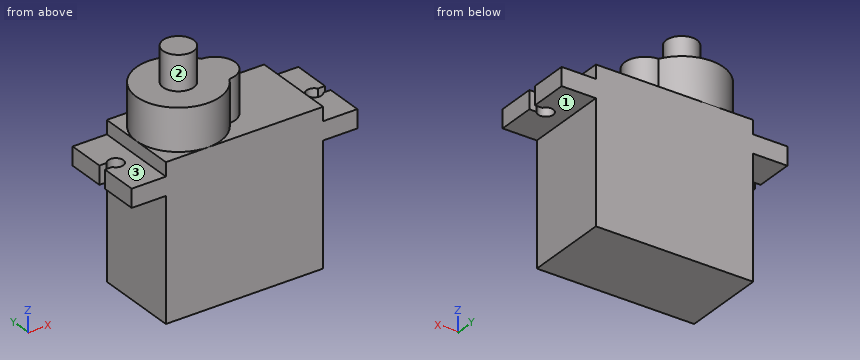
```python
from build123d import *

# Parameters (mm, degrees)
SKETCH2_W           = 23
SKETCH2_H           = 12.3
BOSS_EXTRUDE1_DEPTH = 22.4
SKETCH3_W           = 2.67
SKETCH3_H           = 12.3
BOSS_EXTRUDE2_DEPTH = 5
CUT_EXTRUDE1_DEPTH  = 27.948701267
BOSS_EXTRUDE3_DEPTH = 6.13
SKETCH5_R           = 2.25
BOSS_EXTRUDE4_DEPTH = 5.05


with BuildPart() as part:
    # Sketch2 → Boss-Extrude1 (new body)
    with BuildSketch(Plane.XY):
        Rectangle(SKETCH2_W, SKETCH2_H)
    extrude(amount=BOSS_EXTRUDE1_DEPTH)

    # Sketch3 → Boss-Extrude2 (add)
    with BuildSketch(Plane(origin=(11.5, 0, 0), x_dir=(0, 0, -1), z_dir=(1, 0, 0))):
        with Locations((-19.065, 0)):
            Rectangle(SKETCH3_W, SKETCH3_H)
    boss_extrude2 = extrude(amount=BOSS_EXTRUDE2_DEPTH)

    # Sketch6 → Cut-Extrude1 (cut, through all)
    with BuildSketch(Plane.XY.offset(20.4)):
        with BuildLine():
            Line((15.437749967, 0.575), (16.5, 0.575))
            Line((16.5, 0.575), (16.5, -0.575))
            Line((16.5, -0.575), (15.437749967, -0.575))
            ThreePointArc((15.437749967, -0.575), (13.4, 0), (15.437749967, 0.575))
        make_face()
    cut_extrude1 = extrude(amount=-CUT_EXTRUDE1_DEPTH, mode=Mode.SUBTRACT)

    # Mirror1: Boss-Extrude2, Cut-Extrude1 across plane
    add(boss_extrude2.mirror(Plane(origin=(0, 0, 0), x_dir=(0, 0, 1), z_dir=(1, 0, 0))))
    add(cut_extrude1.mirror(Plane(origin=(0, 0, 0), x_dir=(0, 0, 1), z_dir=(1, 0, 0))), mode=Mode.SUBTRACT)

    # Sketch4 → Boss-Extrude3 (add)
    with BuildSketch(Plane.XY.offset(22.4)):
        with BuildLine():
            ThreePointArc((0.060221963, 2.924379988), (-11.5, 0), (0.060221963, -2.924379988))
            ThreePointArc((0.060221963, -2.924379988), (2.925, 0), (0.060221963, 2.924379988))
        make_face()
    extrude(amount=BOSS_EXTRUDE3_DEPTH)

    # Sketch5 → Boss-Extrude4 (add)
    with BuildSketch(Plane.XY.offset(28.53)):
        with Locations((-5.35, 0)):
            Circle(SKETCH5_R)
    extrude(amount=BOSS_EXTRUDE4_DEPTH)


solid = part.part
```
Input: part model. Units: mm. Frame: model coordinates. Face numbers are marked on the shaded views. A direction names the side the tool comes from. Coordinates: 2 decimals unless noted, no trailing zeros. Loops run counter-clockwise (first coordinate to the right, second up) from the corner with the lowest first, then second, coordinate; pieces in that order, holes last.
Q1. Section D-D, the plane z = 2.5. Return the cut outline in (x, y).
Results are:
outline: (-11.5, -6.15) - (11.5, -6.15) - (11.5, 6.15) - (-11.5, 6.15) - close
Q2. Line query: line 1 along Y through (x, z) = (-14.5, 18.3); line 2 along Z through (x, y) = (-9.5, 1.25); line 3 along X through (y, z) = (0, 18.75). Output: solid intervals per line, ascending.
Results are:
line 1: y = -6.15 to -1.1, 1.1 to 6.15
line 2: z = 0 to 28.53
line 3: x = -13.4 to 13.4
Q3. Section B-B, the plane y = -4. Return the cut outline in (x, z).
Results are:
outline: (-16.5, 17.73) - (-11.5, 17.73) - (-11.5, 0) - (11.5, 0) - (11.5, 17.73) - (16.5, 17.73) - (16.5, 20.4) - (11.5, 20.4) - (11.5, 22.4) - (-0.68, 22.4) - (-0.68, 28.53) - (-10.02, 28.53) - (-10.02, 22.4) - (-11.5, 22.4) - (-11.5, 20.4) - (-16.5, 20.4) - close
Q4. Contact query for flat-ended pins moving along their axis: pin 1 (2.5 mm diameter, centred on x = -13, y = -2, fed in from +Z); pin 2 (4 mm diameter, centred on y = -4.5, z = 8, fed in from -X); pin 3 (3 mm diameter, centred on x = -9.5, y = -3.5, fed in from +Z); pin 4 (1.8 mm diameter, centred on x = -14.5, y = 0, fed in from +Z). Output: stop coordinate, or through.
Results are:
pin 1: stops at z = 20.4
pin 2: stops at x = -11.5
pin 3: stops at z = 28.53
pin 4: passes through
Q5. Set-up query: the marked faces 1, 2 and 3. Return all of +Z, -Z, +X, -X, +Y, -Y with unobstructed straight access to the full face (end or side cutting, diameter ignored); none if empty.
Results are:
face 1: -Z, +X, +Y, -Y
face 2: +Z
face 3: +Z, -X, +Y, -Y
Q6. Section A-A, the plane x = 14.5. Return the cut outline in (y, z).
Results are:
outline: (-6.15, 17.73) - (-1.1, 17.73) - (-1.1, 20.4) - (-6.15, 20.4) - close; (1.1, 17.73) - (6.15, 17.73) - (6.15, 20.4) - (1.1, 20.4) - close
Q7. Section C-C, the plane x = -1.5. Return the cut outline in (y, z).
Results are:
outline: (-6.15, 0) - (6.15, 0) - (6.15, 22.4) - (4.8, 22.4) - (4.8, 28.53) - (-4.8, 28.53) - (-4.8, 22.4) - (-6.15, 22.4) - close
